```python
from build123d import *

# Parameters (mm, degrees)
ESTRUSIONE_ESTRUSIONE1_DEPTH = 150
TAGLIO_ESTRUSIONE1_DEPTH     = 145


with BuildPart() as part:
    # Schizzo2 → Estrusione-Estrusione1 (new body)
    with BuildSketch(Plane(origin=(0, 0, 0), x_dir=(1, 0, 0), z_dir=(0, 1, 0))):
        Polygon((19, 96), (19, 87), (26, 87), (26, 91), (34, 91), (34, 76), (26, 76), (26, 80), (19, 80), (19, 0), (0, 0), (0, 96), align=None)
    extrude(amount=ESTRUSIONE_ESTRUSIONE1_DEPTH)

    # Schizzo3 → Taglio-Estrusione1 (cut)
    with BuildSketch(Plane.XZ):
        with BuildLine():
            Line((8.958039892, -91), (5, -91))
            Line((5, -91), (5, -74))
            Line((5, -74), (8.958039892, -74))
            ThreePointArc((8.958039892, -74), (15, -82.5), (8.958039892, -91))
        make_face()
    extrude(amount=-TAGLIO_ESTRUSIONE1_DEPTH, mode=Mode.SUBTRACT)

    # Specchia2: part across plane


with BuildPart() as part_1:
    add(part.part)
    add(part.part.mirror(Plane(origin=(19, 150, 0), x_dir=(1, 0, 0), z_dir=(0, 0, -1))))


solid = part_1.part
```
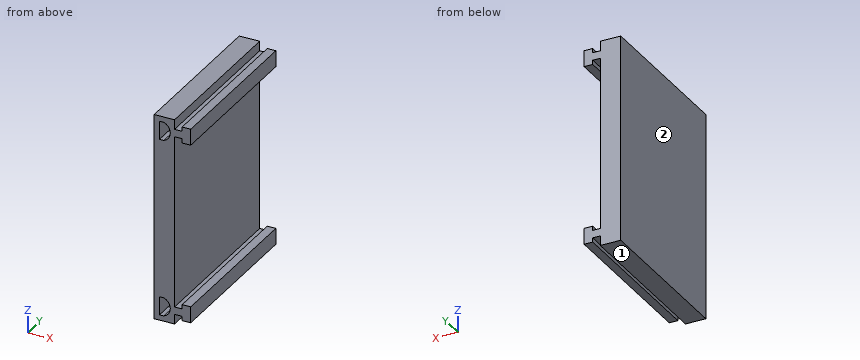
Verification items for the finished model (mm, model axes). Face numbers are marked on the shaded views. Give positions to 0.01 mm unless a question says otherwise; leave off trailing zeros. Order: outer loops, then holes, each group sorted by start corner. A loop starts at its lowest first (then second) coordinate and runs counter-clockwise, first axis right, second up. Notation, with made-up numbers: M 5,37 L 34,37 A31 ccw 34,74 Z; hole C 23,39.5 d4. An arc over 180 degrees is marked long. Return JSON: item names as keys, results as strings. Group by question number.
1) Scan lines: line 1 (Z direction, x = 5.5, y = 119); line 2 (Z direction, x = 29, y = 37); line 3 (Z direction, x = 20, y = 87). Record each from-to range of solid material in increasing order.
2) Section check B-B on y = 86.5. Record the cut outline in (x, z), and give its area (3 significant figures).
3) Go/stop test with flat-tipped pins: pin 1 Ø4 at (x, y) = (31, 54.5) entering from -Z; pin 2 Ø7.5 at (x, y) = (24, 99.5) entering from +Z; pin 3 Ø3.5 at (x, y) = (21, 94.5) entering from -Z. Record where each tip stops, or that it passes through.
4) Mould release check, pull along X, two halves, no side actions. Record for the marked faces 1 and 2: pulls with the +X half, pulls with the -X half, needs draft (parallel to the pull), parting line crosses it, or undercut.
5) Section check C-C on z = -68.5. Record the cut outline in (x, y), and give its area (3 significant figures).
6) Section check A-A on x = 28. Record the cut outline in (y, z).
Answer block:
{
 "1": {"line 1": "z = -96 to -91, -74 to 74, 91 to 96", "line 2": "z = -91 to -76, 76 to 91", "line 3": "z = -87 to -80, 80 to 87"},
 "2": {"outline": "M 0,-96 L 19,-96 L 19,-87 L 26,-87 L 26,-91 L 34,-91 L 34,-76 L 26,-76 L 26,-80 L 19,-80 L 19,80 L 26,80 L 26,76 L 34,76 L 34,91 L 26,91 L 26,87 L 19,87 L 19,96 L 0,96 Z; hole M 5,-91 L 8.96,-91 A9 ccw 8.96,-74 L 5,-74 Z; hole M 5,74 L 8.96,74 A9 ccw 8.96,91 L 5,91 Z", "area": "3,700 mm^2"},
 "3": {"pin 1": "stops at z = -91", "pin 2": "stops at z = 91", "pin 3": "stops at z = -87"},
 "4": {"face 1": "needs draft", "face 2": "pulls with the -X half"},
 "5": {"outline": "M 0,0 L 19,0 L 19,150 L 0,150 Z", "area": "2,850 mm^2"},
 "6": {"outline": "M 0,-91 L 150,-91 L 150,-76 L 0,-76 Z; M 0,76 L 150,76 L 150,91 L 0,91 Z"}
}
